Autodesk Fusion 360 part; units mm, degrees
sketch "Sketch1" plane through (0, 0, 0) normal (0, 0, 1) x (1, 0, 0)
  circle A0 centre (0, 0) radius 35
  dimension "d6" = 70
extrude "Extrude1" add sketch "Sketch1" along normal blind 100
sketch "Sketch2" plane through (0, 0, 100) normal (0, 0, 1) x (-1, 0, 0)
  circle A0 centre (0, 0) radius 35
  circle A1 centre (0, 0) radius 29.9384
extrude "Extrude2" cut sketch "Sketch2" against normal blind 55 contours A1
fillet "Fillet1" radius 5 1 edges at (-32.6315, -12.6565, 100)
The model under review builds one solid part; all positions refer to its coordinate system, in mm. Give positions to 0.01 mm unless a question says otherwise; leave off trailing zeros. Loops run counter-clockwise (first coordinate to the right, second up) from the corner with the lowest first, then second, coordinate; pieces in that order, holes last. Notation, with made-up numbers: (-6, -19.5) -> (14, -19.5) arc R20 cw to (14, -6.5) -> close; hole circle Ø11 at (67, 26.5). An arc over 180 degrees is marked (long way). Write each question's results on one line, items separated by ' | '.
1) Take a section at D-D, the plane z = 16. Give the boundary of the cut face in (x, y).
Conclusion:
outline: circle Ø70 at (0, 0)
2) Draft analysis for pull direction X (two halves, no side actions). For faces 1 (the face through (-28, 21, 47)), 2 (the face through (0, 0, 0)), 3 (the face through (0, 0, 45)), state which applies: pulls with the +X half, pulls with the -X half, needs draft (parallel to the pull), parting line crosses it, or undercut.
Conclusion:
face 1: parting line crosses it | face 2: needs draft | face 3: undercut
3) Take a section at B-B, the plane z = 60. Give the boundary of the cut face in (x, y), plus the area to 3 significant figures.
Conclusion:
outline: circle Ø70 at (0, 0); hole circle Ø59.88 at (0, 0) | area: 1,030 mm^2
4) Take a section at A-A, the plane y = 0. Give the boundary of the cut face in (x, z), plus the area to 3 significant figures.
Conclusion:
outline: (-35, 0) -> (35, 0) -> (35, 95) arc R5 ccw to (30, 100) -> (29.94, 100) -> (29.94, 45) -> (-29.94, 45) -> (-29.94, 100) -> (-30, 100) arc R5 ccw to (-35, 95) -> close | area: 3,700 mm^2
5) For line 1 along Y through (x, z) = (0, 68.5); line 2 along Z through (x, y) = (-4, -28); line 3 along Y through (x, z) = (-15.5, 94), list the stretches that pass through material, from the lowest coordinate up. Write a range as from..to.
Conclusion:
line 1: y = -35..-29.94, 29.94..35 | line 2: z = 0..45 | line 3: y = -31.38..-25.61, 25.61..31.38
6) Insertion check: pin 1 Ø3 at (x, y) = (-26.5, -18) entering from +Z; pin 2 Ø2 at (x, z) = (12.5, 17.5) entering from -Y; pin 3 Ø3 at (x, z) = (-6, 81.5) entering from +Y. Each pin has a flat end and moves straight along its axis. Give the tip position at first contact, or say it passes through.
Conclusion:
pin 1: stops at z = 99.97 | pin 2: stops at y = -33.06 | pin 3: stops at y = 34.71
